```python
from build123d import *

# Parameters (mm, degrees)
SALIENTE_EXTRUIR1_DEPTH = 1


with BuildPart() as part:
    # Croquis1 → Revolución1 (revolve)
    with BuildSketch(Plane.XY, mode=Mode.PRIVATE) as revoluci_n1_sk:
        with BuildLine():
            Line((0, 40.5), (0, 0))
            ThreePointArc((0, 0), (0.762242399, 0.119036639), (1.451896979, 0.46481078))
            Line((1.451896979, 0.46481078), (5.4, 17))
            Line((5.4, 17), (5.4, 37.5))
            Line((5.4, 37.5), (6.6, 37.5))
            Line((6.6, 37.5), (6.6, 40.5))
            Line((6.6, 40.5), (0, 40.5))
        make_face()
    revolve(revoluci_n1_sk.sketch.rotate(Axis((0, 0, 0), (0, 1, 0)), 180), axis=Axis((0, 0, 0), (0, 1, 0)))

    # Croquis2 → Saliente-Extruir1 (add)
    with BuildSketch(Plane(origin=(0, 40.5, 0), x_dir=(1, 0, 0), z_dir=(0, 1, 0))):
        with BuildLine():
            Line((9.209038218, 3), (2.780130903, 5.985889421))
            ThreePointArc((2.780130903, 5.985889421), (6.6, 0), (2.780130903, -5.985889421))
            Line((2.780130903, -5.985889421), (9.209038218, -3))
            ThreePointArc((9.209038218, -3), (9.685369631, 0), (9.209038218, 3))
        make_face()
    extrude(amount=-SALIENTE_EXTRUIR1_DEPTH)


solid = part.part
```
Model file for the job. Use its own axes, mm. A direction names the side the tool comes from. Round coordinates to 2 decimals unless told otherwise and drop trailing zeros. Write each loop counter-clockwise with the first axis right and the second up, starting at its lowest first coordinate (ties: lowest second). Pieces come first, ordered by that corner, then holes. Notation, with made-up numbers: (8.25, -30) - (32.25, -30) arc R18 cw to (32.25, 1) - close; hole circle Ø11 at (7.5, 17). An arc over 180 degrees is marked (long way). Use CSV: the item, a comma, the result in double quotes. Start each with the question number.
Item 1: Drill centre lines: L1, parallel to Y at x = 7, z = 0.25; L2, parallel to Y at x = 0, z = 5.75; L3, parallel to X at y = 21, z = 2. Where is each one in solid material? Low to high. Write a range as [from, to].
Item 2: Band-saw the part on D-D (y = 14). Write the cut outline in (x, z), and give its area (3 significant figures).
Item 3: Pin check, flat tips, straight feed: P1, Ø6, axis at x = -2, y = 23, coming from the +Z side; P2, Ø4, axis at x = 3, z = 0.5, coming from the -Y side; P3, Ø1, axis at y = 20.5, z = -4, coming from the -X side. Stop position of each tip, or through.
Item 4: Band-saw the part on A-A (x = 0). Write the cut outline in (y, z).
Item 5: Band-saw the part on C-C (y = 21). Write the cut outline in (x, z).
Item 6: Band-saw the part on B-B (z = 0). Write the cut outline in (x, y), and give its area (3 significant figures).
Item 7: Tool access for faces 1 (the face through (6.04, 40.01, -4.47)), 2 (the face through (-6.097, 39.021, -2.528)): list every direction of +Z, -Z, +X, -X, +Y, -Y with a clear straight run to the whole face (end or side of a thin tool).
Checked values:
1,L1,"y = [39.5, 40.5]"
1,L2,"y = [37.5, 40.5]"
1,L3,"x = [-5.02, 5.02]"
2,outline,"circle Ø9.37 at (0, 0)"
2,area,"68.9 mm²"
3,P1,"stops at z = 5.4"
3,P2,"stops at y = 0.23"
3,P3,"stops at x = -4.11"
4,outline,"(0.46, -1.45) - (17, -5.4) - (37.5, -5.4) - (37.5, -6.6) - (40.5, -6.6) - (40.5, 6.6) - (37.5, 6.6) - (37.5, 5.4) - (17, 5.4) - (0.46, 1.45) arc R2.5 ccw to start"
5,outline,"circle Ø10.8 at (0, 0)"
6,outline,"(-6.6, 37.5) - (-5.4, 37.5) - (-5.4, 17) - (-1.45, 0.46) arc R2.5 ccw to (1.45, 0.46) - (5.4, 17) - (5.4, 37.5) - (6.6, 37.5) - (6.6, 39.5) - (9.69, 39.5) - (9.69, 40.5) - (-6.6, 40.5) - close"
6,area,"378 mm²"
7,face 1,"-Z, +X, +Y, -Y"
7,face 2,"-Y"
